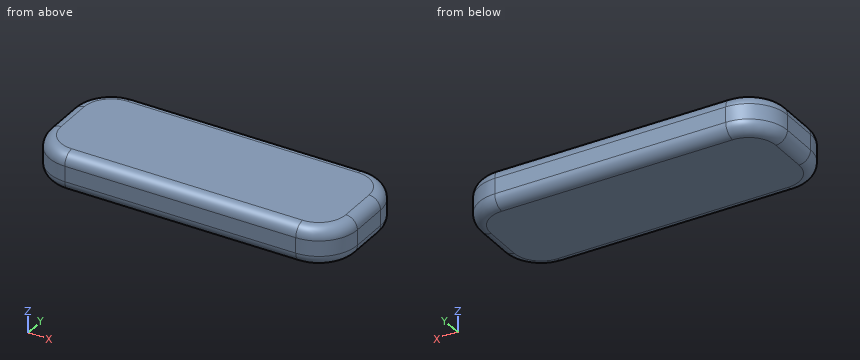
from build123d import *

# Parameters (mm, degrees)
SKETCH_1_W      = 80
SKETCH_1_H      = 30
EXTRUDE_1_DEPTH = 10
FILLET_1_R      = 10
FILLET_3_R      = 3


with BuildPart() as part:
    # 草图1 → 凸台-拉伸1 (new body)
    with BuildSketch(Plane.XY):
        Rectangle(SKETCH_1_W, SKETCH_1_H)
    extrude(amount=EXTRUDE_1_DEPTH)

    # 圆角1
    fillet_1_edges = [part.edges().sort_by_distance(p)[0] for p in [
        (-40, 15, 5),
        (40, 15, 5),
        (40, -15, 5),
        (-40, -15, 5),
    ]]
    fillet(fillet_1_edges, radius=FILLET_1_R)

    # 圆角3
    fillet_3_edges = [part.edges().sort_by_distance(p)[0] for p in [
        (40, 0, 0),
        (40, 0, 10),
        (-40, 0, 0),
        (0, 15, 0),
        (0, -15, 0),
        (-37.071067812, -12.071067812, 0),
        (-37.071067812, 12.071067812, 0),
        (37.071067812, 12.071067812, 0),
        (37.071067812, -12.071067812, 0),
        (0, -15, 10),
        (-40, 0, 10),
        (0, 15, 10),
        (-37.071067812, -12.071067812, 10),
        (-37.071067812, 12.071067812, 10),
        (37.071067812, 12.071067812, 10),
        (37.071067812, -12.071067812, 10),
    ]]
    fillet(fillet_3_edges, radius=FILLET_3_R)


solid = part.part
Build history of the part. All positions in model axes, mm. Give positions to 0.01 mm unless a question says otherwise; leave off trailing zeros. Write each loop counter-clockwise with the first axis right and the second up, starting at its lowest first coordinate (ties: lowest second). Pieces come first, ordered by that corner, then holes. Notation, with made-up numbers: (4.25, -6) - (50.25, -6) arc R16 cw to (50.25, 19) - close; hole circle Ø3 at (-12, -12.5). An arc over 180 degrees is marked (long way). Use one line per item in the form item = value. Start each with the question number.
1. Band-saw the part on A-A on x = -2. Write the cut outline in (y, z).
2. Band-saw the part on B-B on z = 4.25. Write the cut outline in (x, y).
3. Drop a flat-ended pin along its axis: pin 1 Ø5 at (y, z) = (-11, 5.5) entering from +X. Give the stop position or say it passes through.
4. Probe line 1 (X direction, y = -5, z = 2.75); line 2 (Y direction, x = 32.5, z = 7); line 3 (X direction, y = 6.5, z = 3.5). List the from-to ranges inside material, lowest first. Write a range as [from, to].
Conclusion:
q1.outline = (-15, 3) arc R3 ccw to (-12, 0) - (12, 0) arc R3 ccw to (15, 3) - (15, 7) arc R3 ccw to (12, 10) - (-12, 10) arc R3 ccw to (-15, 7) - close
q2.outline = (-40, -5) arc R10 ccw to (-30, -15) - (30, -15) arc R10 ccw to (40, -5) - (40, 5) arc R10 ccw to (30, 15) - (-30, 15) arc R10 ccw to (-40, 5) - close
q3.pin_1 = 39.37
q4.line_1 = [-39.99, 39.99]
q4.line_2 = [-14.68, 14.68]
q4.line_3 = [-39.89, 39.89]
